Design review of the part built by this model. Coordinates are the model's own, in mm. A direction names the side the tool comes from. Round coordinates to 2 decimals unless told otherwise and drop trailing zeros. Loops run counter-clockwise (first coordinate to the right, second up) from the corner with the lowest first, then second, coordinate; pieces in that order, holes last. Notation, with made-up numbers: M 44,-2 L 65,-2 A36 ccw 65,37 Z; hole C -3.75,25 d2. An arc over 180 degrees is marked long. One line per item, written item: value. Start each with the question number.
Item 1: We need section B-B (y = -3.5). Write out the cut boundary in (x, z), then the cut area to 3 significant figures.
Item 2: We need section D-D (x = 25). Write out the cut boundary in (y, z), then the cut area to 3 significant figures.
Item 3: Clearance check with flat-ended pins moving along their axes: pin 1 (1 mm diameter, centred on x = 12, z = 48, fed in from +Y); pin 2 (7 mm diameter, centred on x = 25, y = 25, fed in from -Z); pin 3 (2 mm diameter, centred on x = 29, z = 65, fed in from +Y). State where each tip first meets the part, or that it passes through.
Item 4: For line 1 along Y through (x, z) = (25, 30); line 2 along X through (y, z) = (-25, 170.5); line 3 along X through (y, z) = (15, 106.5), list the stretches that pass through material, from the lowest coordinate up.
Item 5: For faces 4 (the cylindrical face through (-15.1, -19.5, 110.6)), 5 (the flat face through (-30, -24, 106)), list the 3-axis set-ups (+Z, -Z, +X, -X, +Y, -Y) from which the entire face can be reached by the end or side of a thin tool; tool diameter is ignored.
Item 6: We need section C-C (z = 91.5). State how many separate pieces and enclosed holes the cut face has, then the cut area to 3 significant figures.
Item 7: Mouldability with a two-part tool opening along X and no side actions: class faces 1 (the flat face through (30, 0, 116)), 2 (the cylindrical face through (-19.5, -14.9, 111.4)), 3 (the flat face through (0, -30, 106)) as released by +X, released by -X, zero draft, split by the parting line, or undercut.
Item 8: We need section A-A (y = -25). Write out the cut boundary in (x, z), then the cut area to 3 significant figures.
from build123d import *

# Parameters (mm, degrees)
F0_R          = 3
F0_R_2        = 2.5
F1_DEPTH      = 214.17
F2_R          = 2
F3_R          = 7
F5_DEPTH      = 30
F5_DEPTH_BACK = 30


# Not quite as in the source:
# - a feature names something its author has since deleted; it is built from what else it names


with BuildPart() as f1:
    # F0 (on Top) → F1 (new body)
    with BuildSketch(Plane.XY):
        with BuildLine():
            Line((18.15, -30), (30, -30))
            Line((30, -30), (30, -18.15))
            Line((30, -18.15), (27.5, -18.15))
            Line((27.5, -18.15), (27.5, -20.15))
            Line((27.5, -20.15), (21.5477069044, -20.15))
            ThreePointArc((21.5477069044, -20.15), (19.5, -15), (21.5477069044, -9.85))
            Line((21.5477069044, -9.85), (27.5, -9.85))
            Line((27.5, -9.85), (27.5, -11.85))
            Line((27.5, -11.85), (30, -11.85))
            Line((30, -11.85), (30, 11.85))
            Line((30, 11.85), (27.5, 11.85))
            Line((27.5, 11.85), (27.5, 9.85))
            Line((27.5, 9.85), (21.5477069044, 9.85))
            ThreePointArc((21.5477069044, 9.85), (19.5, 15), (21.5477069044, 20.15))
            Line((21.5477069044, 20.15), (27.5, 20.15))
            Line((27.5, 20.15), (27.5, 18.15))
            Line((27.5, 18.15), (30, 18.15))
            Line((30, 18.15), (30, 30))
            Line((30, 30), (18.15, 30))
            Line((18.15, 30), (18.15, 27.5))
            Line((18.15, 27.5), (20.15, 27.5))
            Line((20.15, 27.5), (20.15, 21.5477069044))
            ThreePointArc((20.15, 21.5477069044), (15, 19.5), (9.85, 21.5477069044))
            Line((9.85, 21.5477069044), (9.85, 27.5))
            Line((9.85, 27.5), (11.85, 27.5))
            Line((11.85, 27.5), (11.85, 30))
            Line((11.85, 30), (-11.85, 30))
            Line((-11.85, 30), (-11.85, 27.5))
            Line((-11.85, 27.5), (-9.85, 27.5))
            Line((-9.85, 27.5), (-9.85, 21.5477069044))
            ThreePointArc((-9.85, 21.5477069044), (-15, 19.5), (-20.15, 21.5477069044))
            Line((-20.15, 21.5477069044), (-20.15, 27.5))
            Line((-20.15, 27.5), (-18.15, 27.5))
            Line((-18.15, 27.5), (-18.15, 30))
            Line((-18.15, 30), (-30, 30))
            Line((-30, 30), (-30, 18.15))
            Line((-30, 18.15), (-27.5, 18.15))
            Line((-27.5, 18.15), (-27.5, 20.15))
            Line((-27.5, 20.15), (-21.5477069044, 20.15))
            ThreePointArc((-21.5477069044, 20.15), (-19.5, 15), (-21.5477069044, 9.85))
            Line((-21.5477069044, 9.85), (-27.5, 9.85))
            Line((-27.5, 9.85), (-27.5, 11.85))
            Line((-27.5, 11.85), (-30, 11.85))
            Line((-30, 11.85), (-30, -11.85))
            Line((-30, -11.85), (-27.5, -11.85))
            Line((-27.5, -11.85), (-27.5, -9.85))
            Line((-27.5, -9.85), (-21.5477069044, -9.85))
            ThreePointArc((-21.5477069044, -9.85), (-19.5, -15), (-21.5477069044, -20.15))
            Line((-21.5477069044, -20.15), (-27.5, -20.15))
            Line((-27.5, -20.15), (-27.5, -18.15))
            Line((-27.5, -18.15), (-30, -18.15))
            Line((-30, -18.15), (-30, -30))
            Line((-30, -30), (-18.15, -30))
            Line((-18.15, -30), (-18.15, -27.5))
            Line((-18.15, -27.5), (-20.15, -27.5))
            Line((-20.15, -27.5), (-20.15, -21.5477069044))
            ThreePointArc((-20.15, -21.5477069044), (-15, -19.5), (-9.85, -21.5477069044))
            Line((-9.85, -21.5477069044), (-9.85, -27.5))
            Line((-9.85, -27.5), (-11.85, -27.5))
            Line((-11.85, -27.5), (-11.85, -30))
            Line((-11.85, -30), (11.85, -30))
            Line((11.85, -30), (11.85, -27.5))
            Line((11.85, -27.5), (9.85, -27.5))
            Line((9.85, -27.5), (9.85, -21.5477069044))
            ThreePointArc((9.85, -21.5477069044), (15, -19.5), (20.15, -21.5477069044))
            Line((20.15, -21.5477069044), (20.15, -27.5))
            Line((20.15, -27.5), (18.15, -27.5))
            Line((18.15, -27.5), (18.15, -30))
        make_face()
        with Locations((-25, -25)):
            Circle(F0_R, mode=Mode.SUBTRACT)
        with Locations((-15, -15)):
            Circle(F0_R_2, mode=Mode.SUBTRACT)
        with Locations((25, -25)):
            Circle(F0_R, mode=Mode.SUBTRACT)
        with Locations((15, -15)):
            Circle(F0_R_2, mode=Mode.SUBTRACT)
        with Locations((-25, 25)):
            Circle(F0_R, mode=Mode.SUBTRACT)
        with Locations((-15, 15)):
            Circle(F0_R_2, mode=Mode.SUBTRACT)
        Polygon((-7, 22), (-7, 27.5), (0, 27.5), (7, 27.5), (7, 22), (10, 16), (10, 10), (16, 10), (22, 7), (27.5, 7), (27.5, 0), (27.5, -7), (22, -7), (16, -10), (10, -10), (10, -16), (7, -22), (7, -27.5), (0, -27.5), (-7, -27.5), (-7, -22), (-10, -16), (-10, -10), (-16, -10), (-22, -7), (-27.5, -7), (-27.5, 0), (-27.5, 7), (-22, 7), (-16, 10), (-10, 10), (-10, 16), align=None, mode=Mode.SUBTRACT)
        with Locations((15, 15)):
            Circle(F0_R_2, mode=Mode.SUBTRACT)
        with Locations((25, 25)):
            Circle(F0_R, mode=Mode.SUBTRACT)
    extrude(amount=F1_DEPTH)

    # F2
    f2_edges = [f1.edges().sort_by_distance(p)[0] for p in [
        (-7, 27.5, 107.085),
        (7, 27.5, 107.085),
    ]]
    fillet(f2_edges, radius=F2_R)

    # F3
    f3_edges = [f1.edges().sort_by_distance(p)[0] for p in [
        (-10, 16, 107.085),
        (10, 16, 107.085),
    ]]
    fillet(f3_edges, radius=F3_R)

    # F4 (on Right) → F5 (cut, two sides)
    with BuildSketch(Plane.YZ) as f5_sk:
        Polygon((71.6507620084, 117.7635412378), (-30, 0), (52.6850404625, -71.3718123739), (154.335802471, 46.3917288639), align=None)
    extrude(amount=F5_DEPTH, mode=Mode.SUBTRACT)
    extrude(f5_sk.sketch, amount=-F5_DEPTH_BACK, mode=Mode.SUBTRACT)


solid = f1.part
A:
1. outline: M -30,30.7 L -27.5,30.7 L -27.5,214.17 L -30,214.17 Z; M 27.5,30.7 L 30,30.7 L 30,214.17 L 27.5,214.17 Z
1. area: 917 mm2
2. outline: M -30,0 L -28,2.32 L -28,214.17 L -30,214.17 Z; M -22,9.27 L -20.15,11.41 L -20.15,214.17 L -22,214.17 Z; M -9.85,23.34 L -7,26.65 L -7,214.17 L -9.85,214.17 Z; M 7,42.86 L 9.85,46.17 L 9.85,214.17 L 7,214.17 Z; M 20.15,58.1 L 22,60.24 L 22,214.17 L 20.15,214.17 Z; M 28,67.19 L 30,69.51 L 30,214.17 L 28,214.17 Z
2. area: 2,400 mm2
3. pin 1: y = 11.86
3. pin 2: z = 59.66
3. pin 3: y = 26.97
4. line 1: -30 to -28, -22 to -20.15, -9.85 to -7
4. line 2: -30 to -28, -22 to -20.15, -9.85 to -7, 7 to 9.85, 20.15 to 22, 28 to 30
4. line 3: -19.5 to -17.5, -12.5 to -9.97, 9.97 to 12.5, 17.5 to 19.5
5. face 4: +Z, -Z
5. face 5: +Z, -Z, -X, +Y, -Y
6. separate pieces: 1
6. enclosed holes: 9
6. area: 1,080 mm2
7. face 1: released by +X
7. face 2: undercut
7. face 3: zero draft
8. outline: M -30,5.79 L -28,5.79 L -28,214.17 L -30,214.17 Z; M -22,5.79 L -20.15,5.79 L -20.15,214.17 L -22,214.17 Z; M -9.85,5.79 L -7,5.79 L -7,214.17 L -9.85,214.17 Z; M 7,5.79 L 9.85,5.79 L 9.85,214.17 L 7,214.17 Z; M 20.15,5.79 L 22,5.79 L 22,214.17 L 20.15,214.17 Z; M 28,5.79 L 30,5.79 L 30,214.17 L 28,214.17 Z
8. area: 2,790 mm2
